The figure shows three views and two pictorial views of one solid part (mm, origin at its lowest corner). Answer the questions. Coordinates: 2 decimals unless noted, no trailing zeros. Loops run counter-clockwise (first coordinate to the right, second up) from the corner with the lowest first, then second, coordinate; pieces in that order, holes last. Notation, with made-up numbers: (32, -35) -> (46, -35) arc R15 ccw to (46, -29) -> close; hole circle Ø8 at (-24.5, -21). An arc over 180 degrees is marked (long way). Answer as a JSON object with one key per item and string values. Group by question number.
1) Section A-A, the plane y = 5 is taken. Give the vertices of the cut face in (x, z), plus the area to 4 significant figures.
2) Section B-B, the plane x = 0.9 is taken. Give the vertices of the cut face in (y, z).
3) Section D-D, the plane y = 1.5 is taken. Give the vertices of the cut face in (x, z).
4) Consider probe 1 along Z at (x, y) = (0.85, 5); probe 2 along Y at (x, z) = (0.4, 77.5); probe 3 along Z at (x, y) = (2.8, 4.5). Determine where each line is inside the solid, lowest interval first. Write a range as [from, to].
5) Flat-ended cylindrical pins translate along their axes: P1, Ø1.8, axis at y = 5, z = 77.5, coming from the +X side; P2, Ø1.5, axis at x = 0.5, y = 6, coming from the +Z side. Find the tip coordinate at first contact, or state that the pin passes through.
6) Section C-C, the plane y = 8 is taken. Give the vertices of the cut face in (x, z), plus the area to 4 significant figures.
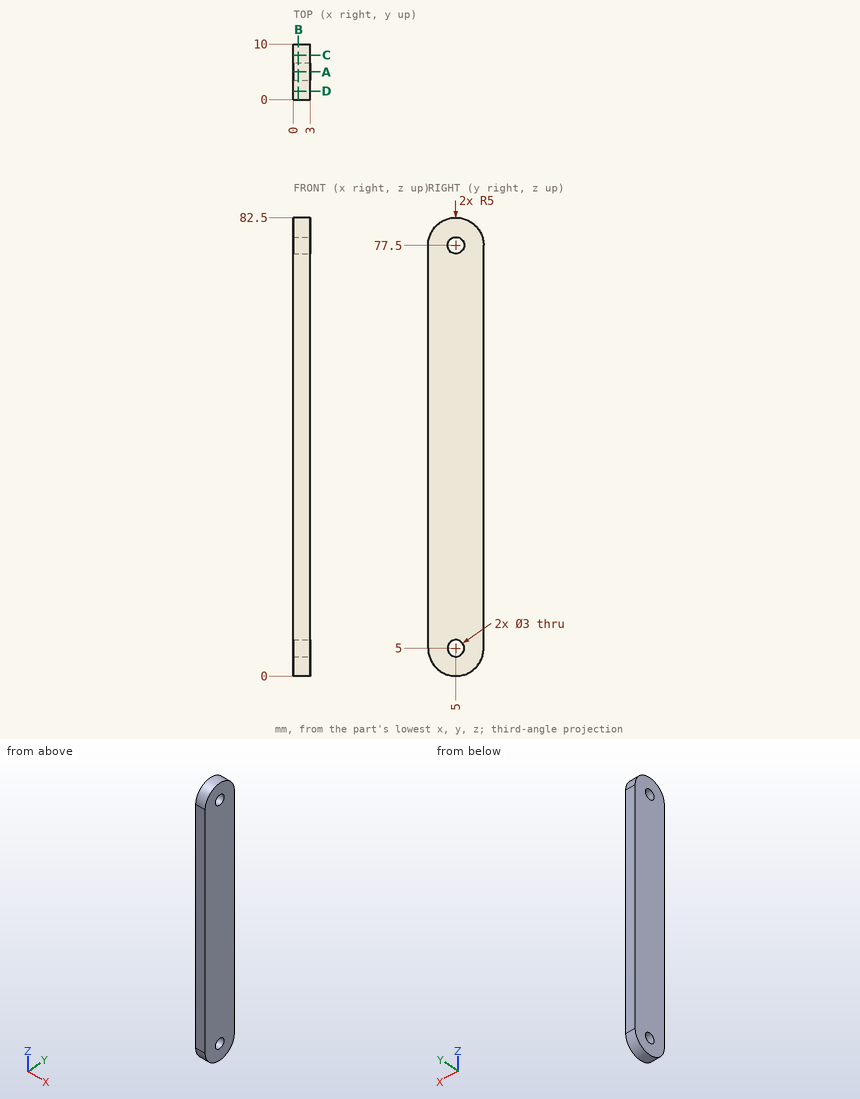
Determined:
{
 "1": {"outline": "(0, 0) -> (3, 0) -> (3, 3.5) -> (0, 3.5) -> close; (0, 6.5) -> (3, 6.5) -> (3, 76) -> (0, 76) -> close; (0, 79) -> (3, 79) -> (3, 82.5) -> (0, 82.5) -> close", "area": "229.5 mm²"},
 "2": {"outline": "(0, 5) arc R5 ccw to (10, 5) -> (10, 77.5) arc R5 ccw to (0, 77.5) -> close; hole circle Ø3 at (5, 5); hole circle Ø3 at (5, 77.5)"},
 "3": {"outline": "(0, 1.43) -> (3, 1.43) -> (3, 81.07) -> (0, 81.07) -> close"},
 "4": {"probe 1": "[0, 3.5], [6.5, 76], [79, 82.5]", "probe 2": "[0, 3.5], [6.5, 10]", "probe 3": "[0.03, 3.59], [6.41, 76.09], [78.91, 82.47]"},
 "5": {"P1": "through", "P2": "z = 82.49"},
 "6": {"outline": "(0, 1) -> (3, 1) -> (3, 81.5) -> (0, 81.5) -> close", "area": "241.5 mm²"}
}
